```python
from build123d import *

# Parameters (mm, degrees)
ESQUISSE1_R        = 6
ESQUISSE1_R_2      = 1.5
BOSS_EXTRU_1_DEPTH = 3


with BuildPart() as part:
    # Esquisse1 → Boss.-Extru.1 (new body)
    with BuildSketch(Plane.XY):
        with Locations((0, 45)):
            Circle(ESQUISSE1_R)
        with Locations((0, 45)):
            Circle(ESQUISSE1_R_2, mode=Mode.SUBTRACT)
        with BuildLine():
            Line((4, 4.472135955), (4, 40.527864045))
            ThreePointArc((4, 40.527864045), (0, 39), (-4, 40.527864045))
            Line((-4, 40.527864045), (-4, 4.472135955))
            ThreePointArc((-4, 4.472135955), (0, 6), (4, 4.472135955))
        make_face()
        Circle(ESQUISSE1_R)
        Circle(ESQUISSE1_R_2, mode=Mode.SUBTRACT)
        with BuildLine():
            Line((-10.382714181, 48.31164637), (-5.880741786, 43.809673974))
            ThreePointArc((-5.880741786, 43.809673974), (-4.242640687, 49.242640687), (1.190326026, 50.880741786))
            Line((1.190326026, 50.880741786), (-3.31164637, 55.382714181))
            ThreePointArc((-3.31164637, 55.382714181), (-4.949747468, 49.949747468), (-10.382714181, 48.31164637))
        make_face()
        with BuildLine():
            ThreePointArc((-12.939033763, 55.593333084), (-6.330461198, 51.397862419), (-10.682211275, 57.904587917))
            Line((-10.682211275, 57.904587917), (-11.115778297, 59.875747229))
            ThreePointArc((-11.115778297, 59.875747229), (-4.955475233, 49.944027426), (-14.870536711, 56.131106542))
            Line((-14.870536711, 56.131106542), (-12.939033763, 55.593333084))
        make_face()
    extrude(amount=BOSS_EXTRU_1_DEPTH)


solid = part.part
```
For this review, take the finished solid that the model builds, in its own axes (mm). A direction names the side the tool comes from. Give positions to 0.01 mm unless a question says otherwise; leave off trailing zeros. Write each loop counter-clockwise with the first axis right and the second up, starting at its lowest first coordinate (ties: lowest second). Pieces come first, ordered by that corner, then holes.
Item 1: Take a section at C-C (x = 0). Give the boundary of the cut face in (y, z).
Item 2: Insertion check: P1, Ø1, axis at x = -1, z = 2.5, coming from the +Y side; P2, Ø1.5, axis at x = 4, z = 1.5, coming from the +Y side. Each pin has a flat end and moves straight along its axis. Give the tip position at first contact, or say it passes through.
Item 3: Machinability: for faces 1 (the face through (4, 22, 1)), 2 (the face through (-10.9, 58.9, 1.5)), 3 (the face through (-13.918, 55.866, 1.479)), 4 (the face through (-0.325, 43.536, 1.479)), 5 (the face through (-1.03, 53.1, 1.48)), which of the approach directions +Z, -Z, +X, -X, +Y, -Y give a long, thin tool a straight path to every point of the face, cutting with its end or side? Answer none if there is none.
Item 4: Take a section at A-A (y = 0). Give the boundary of the cut face in (x, z).
Item 5: Take a section at B-B (z = 2.15). Give the boundary of the cut face in (x, y), and give its area (3 significant figures).
Item 6: The part is to be moulded in two halves that separate along Y. For faces 6 (the face through (-6.44, 51.29, 1.48)), 7 (the face through (-6.261, 59.427, 1.479)), 8 (the face through (0, 28, 3)), say which applies: +Y half, -Y half, draft (parallel to the pull), parting line (faces both ways), or undercut.
Item 7: Take a section at D-D (y = 45). Give the boundary of the cut face in (x, z).
Item 8: Wall thickness on probe 1 along Y at (x, z) = (-1.25, 0.3); probe 2 along X at (y, z) = (7, 0.9); probe 3 along Y at (x, z) = (0, 1.5): over which ranges is each line inside the solid? List them lowest first.
Established:
1. outline: (-6, 0) - (-1.5, 0) - (-1.5, 3) - (-6, 3) - close; (1.5, 0) - (43.5, 0) - (43.5, 3) - (1.5, 3) - close; (46.5, 0) - (52.07, 0) - (52.07, 3) - (46.5, 3) - close
2. P1: stops at y = 53.57
2. P2: stops at y = 50.04
3. face 1: +Z, -Z, +X
3. face 2: +Z, -Z, -X
3. face 3: +Z, -Z, +Y
3. face 4: +Z, -Z
3. face 5: +Z, -Z, +X, +Y
4. outline: (-6, 0) - (-1.5, 0) - (-1.5, 3) - (-6, 3) - close; (1.5, 0) - (6, 0) - (6, 3) - (1.5, 3) - close
5. outline: (-14.87, 56.13) arc R6 ccw to (-10.38, 48.31) - (-5.88, 43.81) arc R6 ccw to (-4, 40.53) - (-4, 4.47) arc R6 ccw (long way) to (4, 4.47) - (4, 40.53) arc R6 ccw to (1.19, 50.88) - (-3.31, 55.38) arc R6 ccw to (-11.12, 59.88) - (-10.68, 57.9) arc R4 cw (long way) to (-12.94, 55.59) - close; hole circle Ø3 at (0, 0); hole circle Ø3 at (0, 45)
5. area: 564 mm2
6. face 6: undercut
6. face 7: +Y half
6. face 8: draft
7. outline: (-7.07, 0) - (-1.5, 0) - (-1.5, 3) - (-7.07, 3) - close; (1.5, 0) - (6, 0) - (6, 3) - (1.5, 3) - close
8. probe 1: y = -5.87 to -0.83, 0.83 to 44.17, 45.83 to 53.32
8. probe 2: x = -4 to 4
8. probe 3: y = -6 to -1.5, 1.5 to 43.5, 46.5 to 52.07
